Design review of the part built by this model. Coordinates are the model's own, in mm. Face numbers are marked on the shaded views. Coordinates: 2 decimals unless noted, no trailing zeros. Loops run counter-clockwise (first coordinate to the right, second up) from the corner with the lowest first, then second, coordinate; pieces in that order, holes last. Notation, with made-up numbers: (-19, 9.5) -> (33, 9.5) arc R18 cw to (33, 42.5) -> close; hole circle Ø3 at (-8.5, -25). An arc over 180 degrees is marked (long way). Answer as a JSON object with one key per item and string values.
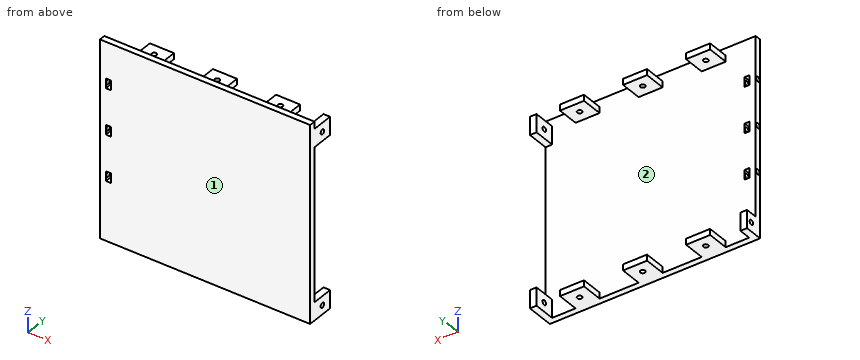
```python
from build123d import *

# Parameters (mm, degrees)
SKETCH1_W               = 175
SKETCH1_H               = 163
BOSS_EXTRUDE1_DEPTH     = 5
SKETCH2_W               = 20
SKETCH2_H               = 5
BOSS_EXTRUDE2_DEPTH     = 18
SKETCH3_R               = 2
CUT_EXTRUDE1_DEPTH      = 7
CUT_EXTRUDE1_DEPTH_BACK = 158
SKETCH4_W               = 5.5
SKETCH4_H               = 15
BOSS_EXTRUDE3_DEPTH     = 18
SKETCH6_W               = 5.5
SKETCH6_H               = 15
BOSS_EXTRUDE4_DEPTH     = 10
SKETCH7_R               = 2
CUT_EXTRUDE3_DEPTH      = 10
SKETCH8_W               = 4.2
SKETCH8_H               = 8
CUT_EXTRUDE4_DEPTH      = 10
SKETCH9_R               = 2
CUT_EXTRUDE5_DEPTH      = 18
SKETCH5_R               = 2
CUT_EXTRUDE8_DEPTH      = 10


with BuildPart() as part:
    # Sketch1 → Boss-Extrude1 (new body)
    with BuildSketch(Plane(origin=(0, 0, 0), x_dir=(1, 0, 0), z_dir=(0, 1, 0))):
        with Locations((-64.046391753, -12.943298969)):
            Rectangle(SKETCH1_W, SKETCH1_H)
    extrude(amount=BOSS_EXTRUDE1_DEPTH)

    # Sketch2 → Boss-Extrude2 (add)
    with BuildSketch(Plane(origin=(0, 5, 0), x_dir=(1, 0, 0), z_dir=(0, 1, 0))):
        with Locations((-116.546391753, 66.056701031)):
            Rectangle(SKETCH2_W, SKETCH2_H)
        with Locations((-116.546391753, -85.943298969)):
            Rectangle(SKETCH2_W, SKETCH2_H)
        with Locations((-11.546391753, -85.943298969)):
            Rectangle(SKETCH2_W, SKETCH2_H)
        with Locations((-11.546391753, 66.056701031)):
            Rectangle(SKETCH2_W, SKETCH2_H)
        with Locations((-64.046391753, -85.943298969)):
            Rectangle(SKETCH2_W, SKETCH2_H)
        with Locations((-64.046391753, 66.056701031)):
            Rectangle(SKETCH2_W, SKETCH2_H)
    extrude(amount=BOSS_EXTRUDE2_DEPTH)

    # Sketch3 → Cut-Extrude1 (cut, two sides)
    with BuildSketch(Plane.XY.offset(88.443298969)) as cut_extrude1_sk:
        with Locations((-116.546391753, 14.1)):
            Circle(SKETCH3_R)
        with Locations((-64.046391753, 14.1)):
            Circle(SKETCH3_R)
        with Locations((-11.546391753, 14.1)):
            Circle(SKETCH3_R)
    extrude(amount=CUT_EXTRUDE1_DEPTH, mode=Mode.SUBTRACT)
    extrude(cut_extrude1_sk.sketch, amount=-CUT_EXTRUDE1_DEPTH_BACK, mode=Mode.SUBTRACT)

    # Sketch4 → Boss-Extrude3 (add)
    with BuildSketch(Plane(origin=(0, 5, 0), x_dir=(1, 0, 0), z_dir=(0, 1, 0))):
        with Locations((-148.796391753, 61.056701031)):
            Rectangle(SKETCH4_W, SKETCH4_H)
        with Locations((-148.796391753, -80.943298969)):
            Rectangle(SKETCH4_W, SKETCH4_H)
    extrude(amount=BOSS_EXTRUDE3_DEPTH)

    # Sketch6 → Boss-Extrude4 (add)
    with BuildSketch(Plane(origin=(0, 5, 0), x_dir=(1, 0, 0), z_dir=(0, 1, 0))):
        with Locations((20.703608247, 61.056701031)):
            Rectangle(SKETCH6_W, SKETCH6_H)
    extrude(amount=BOSS_EXTRUDE4_DEPTH)

    # Sketch7 → Cut-Extrude3 (cut)
    with BuildSketch(Plane(origin=(23.453608247, 0, 0), x_dir=(0, 0, -1), z_dir=(1, 0, 0))):
        with Locations((61.056701031, 10)):
            Circle(SKETCH7_R)
    extrude(amount=-CUT_EXTRUDE3_DEPTH, mode=Mode.SUBTRACT)

    # Sketch8 → Cut-Extrude4 (cut)
    with BuildSketch(Plane(origin=(0, 5, 0), x_dir=(1, 0, 0), z_dir=(0, 1, 0))):
        with Locations((16.353608247, -60.443298969)):
            Rectangle(SKETCH8_W, SKETCH8_H)
        with Locations((16.353608247, -22.443298969)):
            Rectangle(SKETCH8_W, SKETCH8_H)
        with Locations((16.353608247, 15.556701031)):
            Rectangle(SKETCH8_W, SKETCH8_H)
    extrude(amount=-CUT_EXTRUDE4_DEPTH, mode=Mode.SUBTRACT)

    # Sketch9 → Cut-Extrude5 (cut)
    with BuildSketch(Plane(origin=(23.453608247, 0, 0), x_dir=(0, 0, -1), z_dir=(1, 0, 0))):
        with Locations((-22.443298969, 2.5)):
            Circle(SKETCH9_R)
        with Locations((-60.443298969, 2.5)):
            Circle(SKETCH9_R)
        with Locations((15.556701031, 2.5)):
            Circle(SKETCH9_R)
    extrude(amount=-CUT_EXTRUDE5_DEPTH, mode=Mode.SUBTRACT)

    # Sketch5 → Cut-Extrude8 (cut)
    with BuildSketch(Plane(origin=(-146.046391753, 0, 0), x_dir=(0, 0, -1), z_dir=(1, 0, 0))):
        with Locations((61.056701031, 14.1)):
            Circle(SKETCH5_R)
        with Locations((-80.943298969, 14.1)):
            Circle(SKETCH5_R)
    extrude(amount=-CUT_EXTRUDE8_DEPTH, mode=Mode.SUBTRACT)


with BuildPart() as body_2:
    # Mirror3: mirrored copy
    add(part.part.mirror(Plane(origin=(-151.546391753, 5, -68.556701031), x_dir=(0, 0, 1), z_dir=(1, 0, 0))))


solid = body_2.part
```
1) The part is to be moulded in two halves that separate along Z. For the marked faces 1 and 2, say which applies: pulls with the +Z half, pulls with the -Z half, needs draft (parallel to the pull), parting line crosses it, or undercut.
Completed:
{"face 1": "needs draft", "face 2": "undercut"}
2) Add section A-A, the plane y = 19. Count the separate pieces of the cut face and the enclosed holes in it, and give its area (3 significant figures).
Completed:
{"separate pieces": "8", "enclosed holes": "0", "area": "765 mm²"}
3) Add section B-B, the plane x = -193.5. Give the boundary of the cut face in (y, z), and give its area (3 significant figures).
Completed:
{"outline": "(0, -68.56) -> (23, -68.56) -> (23, -63.56) -> (5, -63.56) -> (5, 83.44) -> (23, 83.44) -> (23, 88.44) -> (5, 88.44) -> (5, 94.44) -> (0, 94.44) -> close", "area": "995 mm²"}
4) Clearance check with flat-ended pins moving along their axes: pin 1 Ø3 at (y, z) = (1.5, 21.5) entering from -X; pin 2 Ø10 at (x, z) = (-275.5, 0.5) entering from +Y; pin 3 Ø2.5 at (y, z) = (13, 86.5) entering from -X; pin 4 Ø10 at (x, y) = (-207.5, 11) entering from -Z. State where each tip first meets the part, or that it passes through.
Completed:
{"pin 1": "x = -326.55", "pin 2": "y = 5", "pin 3": "x = -301.55", "pin 4": "through"}
5) Add section C-C, the plane z = -36. Give the boundary of the cut face in (x, y).
Completed:
{"outline": "(-326.55, 0) -> (-151.55, 0) -> (-151.55, 5) -> (-326.55, 5) -> close"}
6) Wall thickness on probe 1 along Z at (x, y) = (-288, 22.25); probe 2 along Y at (x, z) = (-182, -43); probe 3 along X at (y, z) = (8.75, -61): over which ranges is each line inside the solid? List them lowest first.
Completed:
{"probe 1": "-68.56 to -63.56, 83.44 to 88.44", "probe 2": "0 to 5", "probe 3": "-157.05 to -151.55"}
